```python
from build123d import *

# Parameters (mm, degrees)
M5_TAPPED_HOLE1_D       = 4.2
M5_TAPPED_HOLE1_DEPTH   = 12.4
M5_TAPPED_HOLE1_TIP     = 1.2618073
SKETCH5_R               = 42
SKETCH5_R_2             = 32
CUT_EXTRUDE_THIN1_DEPTH = 55.572226802


with BuildPart() as part:
    # Sketch1 → Revolve1 (revolve)
    with BuildSketch(Plane.XY, mode=Mode.PRIVATE) as revolve1_sk:
        with BuildLine():
            Line((-15.404727216, 12), (-15.404727216, 34))
            Line((-15.404727216, 34), (-10.404727216, 34))
            Line((-10.404727216, 34), (-10.404727216, 17))
            Line((-10.404727216, 17), (8.794935567, 17))
            ThreePointArc((8.794935567, 17), (9.450533434, 17.206709213), (9.869004233, 17.752070976))
            Line((9.869004233, 17.752070976), (12.598027216, 25.25))
            Line((12.598027216, 25.25), (15.404727216, 25.25))
            Line((15.404727216, 25.25), (15.404727216, 23.1186))
            Line((15.404727216, 23.1186), (13.829927216, 22.450137059))
            Line((13.829927216, 22.450137059), (13.829927216, 21.187062941))
            Line((13.829927216, 21.187062941), (15.404727216, 20.5186))
            Line((15.404727216, 20.5186), (15.404727216, 12))
            Line((15.404727216, 12), (-15.404727216, 12))
        make_face()
    revolve(revolve1_sk.sketch.rotate(Axis((0, 0, 0), (1, 0, 0)), 90), axis=Axis((0, 0, 0), (1, 0, 0)))

    # M5 Tapped Hole1
    with Locations(Plane.ZY.offset(15.404727216)):
        with Locations((-13.199999999, -22.86307066), (-13.200000001, 22.863070659), (26.4, 1e-09)):
            Hole(M5_TAPPED_HOLE1_D / 2, depth=M5_TAPPED_HOLE1_DEPTH)
            with Locations((0, 0, -(M5_TAPPED_HOLE1_DEPTH + M5_TAPPED_HOLE1_TIP / 2))):  # 118° drill point
                Cone(0, M5_TAPPED_HOLE1_D / 2, M5_TAPPED_HOLE1_TIP, mode=Mode.SUBTRACT)

    # Sketch5 → Cut-Extrude-Thin1 (cut, through all)
    with BuildSketch(Plane(origin=(-10.404727216, 0, 0), x_dir=(0, 0, -1), z_dir=(1, 0, 0))):
        Circle(SKETCH5_R)
        Circle(SKETCH5_R_2, mode=Mode.SUBTRACT)
    extrude(amount=-CUT_EXTRUDE_THIN1_DEPTH, mode=Mode.SUBTRACT)


solid = part.part
```
Part model, mm, in its own coordinate system. A direction names the side the tool comes from. Coordinates: 2 decimals unless noted, no trailing zeros. Write each loop counter-clockwise with the first axis right and the second up, starting at its lowest first coordinate (ties: lowest second). Pieces come first, ordered by that corner, then holes.
Item 1: Slice it at B-B (z = 0). Write the cut outline in (x, y), and give its area (3 significant figures).
Item 2: Slice it at A-A (y = 0). Count the separate pieces of the cut face and the enclosed holes in it, and give its area (3 significant figures).
Item 3: Slice it at C-C (x = 2.5). Write the cut outline in (y, z), and give its area (3 significant figures).
Item 4: Which spindle directions (+Z, -Z, +X, -X, +Y, -Y) get a long thin tool onto all of the face, cutting with end or side? Do faces 4 (the face through (14.02, 15.36, -20.04)), 5 (the face through (-12.87, -31.24, 6.94)), 6 (the face through (-12.87, -21.092, -14.329)), 7 (the face through (-15.405, 14, 0)), 8 (the face through (-0.67, -16.855, -2.213)). Say none if no direction does.
Item 5: Pin check, flat tips, straight feed: pin 1 (8 mm diameter, centred on y = 7, z = 1, fed in from +X); pin 2 (8 mm diameter, centred on x = 11, z = -9, fed in from -Y); pin 3 (3 mm diameter, centred on x = -3, y = 14.5, fed in from -Z); pin 4 (5 mm diameter, centred on x = 10.5, y = 2.5, fed in from +Z). Stop position of each tip, or through.
Item 6: Probe line 1 (Y direction, x = -1.5, z = 0); line 2 (Y direction, x = -5, z = 2); line 3 (Y direction, x = -12.5, z = -13.2). List the from-to ranges inside material, lowest first.
Item 7: Mould opens along Y. For faces 1 (the face through (15.405, 20.5, 11.1)), 2 (the face through (10.04, 16.17, 8.41)), 3 (the face through (-12.87, 0.631, 24.397)) say: released by +Y, released by -Y, zero draft, split by the parting line, or undercut.
Results found:
1. outline: (-15.4, -32) - (-10.4, -32) - (-10.4, -17) - (8.79, -17) arc R1.14 cw to (9.87, -17.75) - (12.6, -25.25) - (15.4, -25.25) - (15.4, -23.12) - (13.83, -22.45) - (13.83, -21.19) - (15.4, -20.52) - (15.4, -12) - (-15.4, -12) - close; (-15.4, 12) - (15.4, 12) - (15.4, 20.52) - (13.83, 21.19) - (13.83, 22.45) - (15.4, 23.12) - (15.4, 25.25) - (12.6, 25.25) - (9.87, 17.75) arc R1.14 cw to (8.79, 17) - (-10.4, 17) - (-10.4, 32) - (-15.4, 32) - close
1. area: 523 mm2
2. separate pieces: 3
2. enclosed holes: 0
2. area: 502 mm2
3. outline: circle Ø34 at (0, 0); hole circle Ø24 at (0, 0)
3. area: 456 mm2
4. face 4: +X
4. face 5: +X, -X
4. face 6: -X
4. face 7: +Z, -Z, -X, +Y, -Y
4. face 8: none
5. pin 1: passes through
5. pin 2: stops at y = -24.68
5. pin 3: stops at z = -10.95
5. pin 4: stops at z = 25.22
6. line 1: y = -17 to -12, 12 to 17
6. line 2: y = -16.88 to -11.83, 11.83 to 16.88
6. line 3: y = -29.15 to -24.96, -20.76 to 20.76, 24.96 to 29.15
7. face 1: zero draft
7. face 2: split by the parting line
7. face 3: undercut
